Input: part model. Units: mm. Frame: model coordinates. Round coordinates to 2 decimals unless told otherwise and drop trailing zeros. Loops run counter-clockwise (first coordinate to the right, second up) from the corner with the lowest first, then second, coordinate; pieces in that order, holes last. Notation, with made-up numbers: (-40, 32) -> (6, 32) arc R15 ccw to (6, 39) -> close; hole circle Ø3 at (70, -20). An arc over 180 degrees is marked (long way). Answer in a Markdown table with one row per item. Add a question column.
Q1. Mould query, pull axis Y, two halves, no side actions, for faces 1 (the face through (37, 3, 23)), 2 (the face through (40, 18, 22)), 3 (the face through (19.19, 21.34, 22.82)), 4 (the face through (20, 36, 22)). Classes: pulls with the +Y half, pulls with the -Y half, needs draft (parallel to the pull), parting line crosses it, or undercut.
Q2. Section C-C, the plane x = 20. Output: boundary loops of the cut face in (y, z).
Q3. Section D-D, the plane y = 32. Output: boundary loops of the cut face in (x, z), and give its area (3 significant figures).
Q4. Section A-A, the plane y = 25. Output: boundary loops of the cut face in (x, z), and give its area (3 significant figures).
Q5. Ray query, L1, parallel to Y at x = 20, z = 27; L2, parallel to X at y = 24, z = 13; L3, parallel to X at y = 25.5, z = 11.5. Return the intervals inside material, ascending. Write a range as from..to.
Q6. Section B-B, the plane z = 5. Output: boundary loops of the cut face in (x, y).
Autodesk Inventor part; units mm, degrees
ref_plane "YZ Plane" through (0, 0, 0) normal (1, 0, 0) x (0, 1, 0)
ref_plane "XZ Plane" through (0, 0, 0) normal (0, 1, 0) x (-1, 0, 0)
ref_plane "XY Plane" through (0, 0, 0) normal (0, 0, 1) x (1, 0, 0)
sketch "Sketch1" plane through (0, 0, 0) normal (0, 0, 1) x (1, 0, 0)
  line L0 (0, 0) -> (40, 0)
  line L1 (40, 0) -> (40, 36)
  line L2 (40, 36) -> (0, 36)
  line L3 (0, 36) -> (0, 0)
  dimension "d0" = 40
  dimension "d1" = 36
extrude "Extrusion1" add sketch "Sketch1" along normal blind 45
sketch "Sketch2" plane through (0, 0, 45) normal (0, 0, 1) x (1, 0, 0)
  circle A0 centre (20, 25) radius 3.75
  line L0 (0, 0) -> (40, 0)
  dimension "d4" = 7.5
  dimension "d7" = 25
extrude "Extrusion2" cut sketch "Sketch2" against normal through all
chamfer "Chamfer1" distance 6 angle 45 4 edges at (40, 36, 22.5) (40, 0, 22.5) (0, 36, 22.5) (0, 0, 22.5)
properties part number "5cm block"
Answer block:
| question | item | result |
|---|---|---|
| 1 | face 1 | pulls with the -Y half |
| 1 | face 2 | needs draft |
| 1 | face 3 | undercut |
| 1 | face 4 | pulls with the +Y half |
| 2 | outline | (0, 0) -> (21.25, 0) -> (21.25, 45) -> (0, 45) -> close; (28.75, 0) -> (36, 0) -> (36, 45) -> (28.75, 45) -> close |
| 3 | outline | (2, 0) -> (38, 0) -> (38, 45) -> (2, 45) -> close |
| 3 | area | 1,620 mm^2 |
| 4 | outline | (0, 0) -> (16.25, 0) -> (16.25, 45) -> (0, 45) -> close; (23.75, 0) -> (40, 0) -> (40, 45) -> (23.75, 45) -> close |
| 4 | area | 1,460 mm^2 |
| 5 | L1 | 0..21.25, 28.75..36 |
| 5 | L2 | 0..16.39, 23.61..40 |
| 5 | L3 | 0..16.28, 23.72..40 |
| 6 | outline | (0, 6) -> (6, 0) -> (34, 0) -> (40, 6) -> (40, 30) -> (34, 36) -> (6, 36) -> (0, 30) -> close; hole circle Ø7.5 at (20, 25) |
